Read the model definition and answer for the solid it produces. Units are mm, in the model's axes. Face numbers are marked on the shaded views. Give positions to 0.01 mm unless a question says otherwise; leave off trailing zeros. Write each loop counter-clockwise with the first axis right and the second up, starting at its lowest first coordinate (ties: lowest second). Pieces come first, ordered by that corner, then holes. Notation, with made-up numbers: M 84.5,53 L 132.5,53 A34 cw 132.5,92 Z; hole C -33.75,81 d10. An arc over 180 degrees is marked long. Use a Markdown table: item, result. Add a question column.
Item 1: A cutting plane is placed at C-C on y = -6. Determine the outline of the cut face in (x, z), then the cut area to 3 significant figures.
Item 2: The mould has two halves that part along Z. Classify the marked faces 1, 2, 3 and 4: pulls with the +Z half, pulls with the -Z half, needs draft (parallel to the pull), parting line crosses it, or undercut.
Item 3: A cutting plane is placed at B-B on x = 0. Determine the outline of the cut face in (y, z), then the cut area to 3 significant figures.
Item 4: A cutting plane is placed at A-A on z = 0. Determine the outline of the cut face in (x, y).
Item 5: A cutting plane is placed at D-D on z = 37.5. Count the separate pieces of the cut face and the enclosed holes in it, then the cut area to 3 significant figures.
Item 6: Given P1, Ø1.5, axis at y = -5.5, z = 71, coming from the -X side; P2, Ø8, axis at x = 33.5, y = 0, coming from the -Z side; P3, Ø8, axis at y = -1.5, z = -19, coming from the +X side, each flat-ended and moving along its own axis, determine where each tip first touches the part or whether it passes through.
Item 7: Consider probe 1 along X at (y, z) = (3.25, 37.5); probe 2 along X at (y, z) = (3.25, 0); probe 3 along Z at (x, y) = (-2, -11.25) (3 decimals). Determine where each line is inside the solid, lowest interval first. Write a range as [from, to].
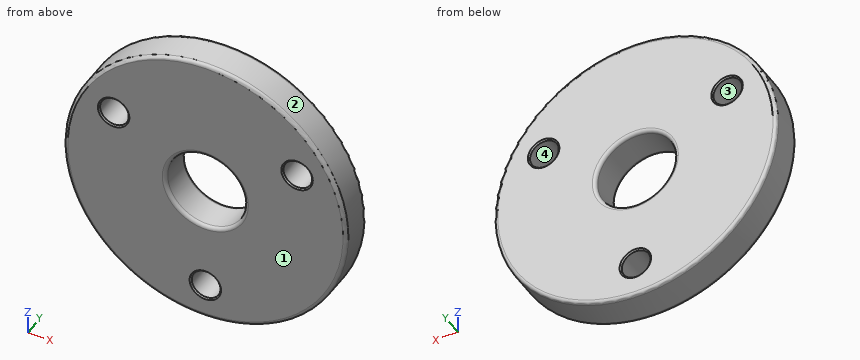
from build123d import *

# Parameters (mm, degrees)
SKETCH1_R           = 100
SKETCH1_R_2         = 28
SKETCH1_R_3         = 10.15
BOSS_EXTRUDE1_DEPTH = 12.5
FILLET1_R           = 2.5
CHAMFER1_SIZE       = 1


with BuildPart() as part:
    # Sketch1 → Boss-Extrude1 (new, symmetric)
    with BuildSketch(Plane(origin=(0, 0, 0), x_dir=(1, 0, 0), z_dir=(0, 1, 0))):
        with Locations(Location((0, 0, 0), (0, 0, 270))):
            Circle(SKETCH1_R)
        with Locations(Location((0, 0, 0), (0, 0, 270))):
            Circle(SKETCH1_R_2, mode=Mode.SUBTRACT)
        with Locations(Location((0, 75, 0), (0, 0, 270))):
            Circle(SKETCH1_R_3, mode=Mode.SUBTRACT)
        with Locations(Location((64.951905284, -37.5, 0), (0, 0, 270))):
            Circle(SKETCH1_R_3, mode=Mode.SUBTRACT)
        with Locations(Location((-64.951905284, -37.5, 0), (0, 0, 270))):
            Circle(SKETCH1_R_3, mode=Mode.SUBTRACT)
    extrude(amount=BOSS_EXTRUDE1_DEPTH, both=True)

    # Fillet1
    fillet1_edges = [part.edges().sort_by_distance(p)[0] for p in [
        (0, -12.5, -100),
        (0, 12.5, -100),
        (0, -12.5, -28),
        (0, 12.5, -28),
    ]]
    fillet(fillet1_edges, radius=FILLET1_R)

    # Chamfer1
    chamfer1_edges = [part.edges().sort_by_distance(p)[0] for p in [
        (64.951905284, -12.5, 27.35),
        (64.951905284, 12.5, 27.35),
        (-64.951905284, -12.5, 27.35),
        (-64.951905284, 12.5, 27.35),
        (0, -12.5, -85.15),
        (0, 12.5, -85.15),
    ]]
    chamfer(chamfer1_edges, length=CHAMFER1_SIZE)


solid = part.part
Filled in:
| question | item | result |
|---|---|---|
| 1 | outline | C 0,0 d200; hole C -64.95,37.5 d20.3; hole C 0,0 d56; hole C 0,-75 d20.3; hole C 64.95,37.5 d20.3 |
| 1 | area | 28,000 mm² |
| 2 | face 1 | needs draft |
| 2 | face 2 | parting line crosses it |
| 2 | face 3 | undercut |
| 2 | face 4 | undercut |
| 3 | outline | M -12.5,-97.5 A2.5 ccw -10,-100 L 10,-100 A2.5 ccw 12.5,-97.5 L 12.5,-86.15 L 11.5,-85.15 L -11.5,-85.15 L -12.5,-86.15 Z; M -12.5,-63.85 L -11.5,-64.85 L 11.5,-64.85 L 12.5,-63.85 L 12.5,-30.5 A2.5 ccw 10,-28 L -10,-28 A2.5 ccw -12.5,-30.5 Z; M -12.5,30.5 A2.5 ccw -10,28 L 10,28 A2.5 ccw 12.5,30.5 L 12.5,97.5 A2.5 ccw 10,100 L -10,100 A2.5 ccw -12.5,97.5 Z |
| 3 | area | 3,080 mm² |
| 4 | outline | M -100,-10 A2.5 ccw -97.5,-12.5 L -30.5,-12.5 A2.5 ccw -28,-10 L -28,10 A2.5 ccw -30.5,12.5 L -97.5,12.5 A2.5 ccw -100,10 Z; M 28,-10 A2.5 ccw 30.5,-12.5 L 97.5,-12.5 A2.5 ccw 100,-10 L 100,10 A2.5 ccw 97.5,12.5 L 30.5,12.5 A2.5 ccw 28,10 Z |
| 5 | separate pieces | 3 |
| 5 | enclosed holes | 0 |
| 5 | area | 3,610 mm² |
| 6 | P1 | x = -71.17 |
| 6 | P2 | z = -95.55 |
| 6 | P3 | x = 98.87 |
| 7 | probe 1 | [-92.7, -75.1], [-54.8, 54.8], [75.1, 92.7] |
| 7 | probe 2 | [-100, -28], [28, 100] |
| 7 | probe 3 | [-99.645, -84.951], [-65.049, -28.264], [28.264, 99.645] |
